Source: CAD feature listing. Evaluate the final solid. Frame: model axes, mm. Face numbers are marked on the shaded views. Give positions to 0.01 mm unless a question says otherwise; leave off trailing zeros. Order: outer loops, then holes, each group sorted by start corner. A loop starts at its lowest first (then second) coordinate and runs counter-clockwise, first axis right, second up.
from build123d import *

# Parameters (mm, degrees)
SKETCH_1_R               = 32
SKETCH_1_R_2             = 23
EXTRUDE_1_DEPTH          = 5
SKETCH_2_R               = 24
CUT_EXTRUDE_1_DEPTH      = 10
PATTERN_CIRCULAR_1_COUNT = 6
SKETCH_3_R               = 1.6
CUT_EXTRUDE_2_DEPTH      = 10
PATTERN_CIRCULAR_2_COUNT = 6
FILLET_1_R               = 3


with BuildPart() as part:
    # 草图1 → 凸台-拉伸1 (new body)
    with BuildSketch(Plane.XY):
        Circle(SKETCH_1_R)
        Circle(SKETCH_1_R_2, mode=Mode.SUBTRACT)
    extrude(amount=EXTRUDE_1_DEPTH)

    # 草图2 → 切除-拉伸1 (cut)
    with BuildSketch(Plane.XY.offset(5)):
        with Locations((0, 50)):
            Circle(SKETCH_2_R)
    cut_extrude_1 = extrude(amount=-CUT_EXTRUDE_1_DEPTH, mode=Mode.SUBTRACT)

    # 阵列(圆周)1: 切除-拉伸1 ×6 about axis
    pattern_circular_1_axis = Axis((0, 0, 0), (0, 0, 1))
    for i in range(1, PATTERN_CIRCULAR_1_COUNT):
        add(cut_extrude_1.rotate(pattern_circular_1_axis, i * 360 / PATTERN_CIRCULAR_1_COUNT), mode=Mode.SUBTRACT)

    # 草图3 → 切除-拉伸2 (cut)
    with BuildSketch(Plane.XY.offset(5)):
        with Locations((13.75, 23.815698604)):
            Circle(SKETCH_3_R)
    cut_extrude_2 = extrude(amount=-CUT_EXTRUDE_2_DEPTH, mode=Mode.SUBTRACT)

    # 阵列(圆周)2: 切除-拉伸2 ×6 about axis
    pattern_circular_2_axis = Axis((0, 0, 0), (0, 0, 1))
    for i in range(1, PATTERN_CIRCULAR_2_COUNT):
        add(cut_extrude_2.rotate(pattern_circular_2_axis, i * 360 / PATTERN_CIRCULAR_2_COUNT), mode=Mode.SUBTRACT)

    # 圆角1
    fillet_1_edges = [part.edges().sort_by_distance(p)[0] for p in [
        (-12.447071945, 29.48, 2.5),
        (12.447071945, 29.48, 2.5),
        (-31.753964876, 3.960519493, 2.5),
        (-19.306892931, 25.519480507, 2.5),
        (19.306892931, 25.519480507, 2.5),
        (31.753964876, 3.960519493, 2.5),
        (31.753964876, -3.960519493, 2.5),
        (19.306892931, -25.519480507, 2.5),
        (-19.306892931, -25.519480507, 2.5),
        (-31.753964876, -3.960519493, 2.5),
        (12.447071945, -29.48, 2.5),
        (-12.447071945, -29.48, 2.5),
    ]]
    fillet(fillet_1_edges, radius=FILLET_1_R)


solid = part.part
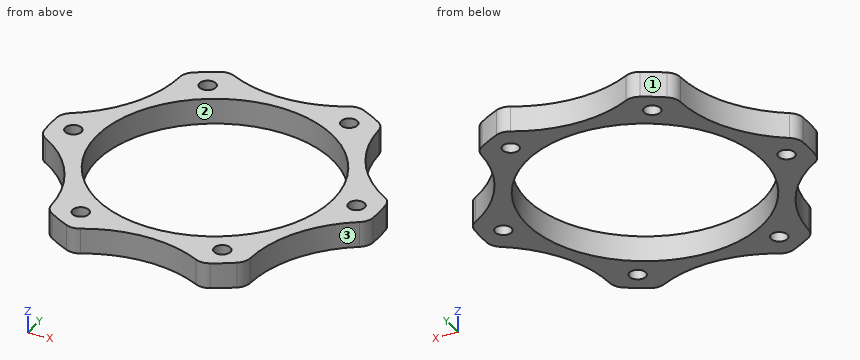
1) First-contact query: pin 1 Ø10 at (x, y) = (11, -9) entering from -Z; pin 2 Ø1.5 at (y, z) = (5, 3.5) entering from -X. Flat tips, straight axial feed; report the tip coordinate or a pass-through.
Checks:
pin 1: passes through
pin 2: stops at x = -31.06
2) Section query D-D on z = 2.2. State how many separate pieces and enclosed holes the cut face has, and give its area (3 significant figures).
Checks:
separate pieces: 1
enclosed holes: 7
area: 898 mm2
3) Ray query, L1, parallel to Y at x = -13.75, z = 1.95; L2, parallel to X at y = 1, z = 3.85; L3, parallel to X at y = -19.5, z = 4.25. Return the intervals inside material, ascending.
Checks:
L1: y = -28.89 to -25.42, -22.22 to -18.44, 18.44 to 22.22, 25.42 to 28.89
L2: x = -31.98 to -28.75, -26.25 to -22.98, 22.98 to 26.25, 28.75 to 31.98
L3: x = -19.94 to -12.2, 12.2 to 19.94
4) Section query C-C on y = -9. Output: boundary loops of the cut face in (x, z).
Checks:
outline: (-25.41, 0) - (-21.17, 0) - (-21.17, 5) - (-25.41, 5) - close; (21.17, 0) - (25.41, 0) - (25.41, 5) - (21.17, 5) - close
5) Section query A-A on y = 0. Output: boundary loops of the cut face in (x, z), and give its area (3 significant figures).
Checks:
outline: (-32, 0) - (-29.1, 0) - (-29.1, 5) - (-32, 5) - close; (-25.9, 0) - (-23, 0) - (-23, 5) - (-25.9, 5) - close; (23, 0) - (25.9, 0) - (25.9, 5) - (23, 5) - close; (29.1, 0) - (32, 0) - (32, 5) - (29.1, 5) - close
area: 58.0 mm2
6) Section query B-B on x = 0. Output: boundary loops of the cut face in (y, z).
Checks:
outline: (-26, 0) - (-23, 0) - (-23, 5) - (-26, 5) - close; (23, 0) - (26, 0) - (26, 5) - (23, 5) - close
7) Pull-direction query (X, two-part tool) for the marked faces 1, 2 and 3; classes: +X half, -X half, draft (parallel to the pull), parting line (faces both ways), or undercut.
Checks:
face 1: -X half
face 2: undercut
face 3: +X half
